```python
from build123d import *

# Parameters (mm, degrees)
SKETCH_1_W          = 35.7
SKETCH_1_H          = 25
EXTRUDE_1_DEPTH     = 1
SKETCH_2_W          = 48
SKETCH_2_H          = 14
EXTRUDE_2_DEPTH     = 57.5
FILLET_1_R          = 3
FILLET_2_R          = 5
CHAMFER_1_SIZE      = 5
HOLE_WIZARD_M3_1_D  = 3.2
CUT_EXTRUDE_START   = -15
CUT_EXTRUDE_1_DEPTH = 15
SKETCH_6_W          = 2
SKETCH_6_H          = 2
EXTRUDE_3_DEPTH     = 8
SKETCH_7_W          = 2
SKETCH_7_H          = 2
SKETCH_7_W_2        = 0.8
SKETCH_7_H_2        = 0.8
CUT_EXTRUDE_2_DEPTH = 6


with BuildPart() as part:
    # 草图1 → 凸台-拉伸1 (new body)
    with BuildSketch(Plane(origin=(0, 0, 0), x_dir=(1, 0, 0), z_dir=(0, 1, 0))):
        Rectangle(SKETCH_1_W, SKETCH_1_H)
    extrude(amount=EXTRUDE_1_DEPTH)

    # 草图2 → 凸台-拉伸2 (add)
    with BuildSketch(Plane(origin=(0, 1, 0), x_dir=(1, 0, 0), z_dir=(0, 1, 0))):
        Rectangle(SKETCH_2_W, SKETCH_2_H)
    extrude(amount=EXTRUDE_2_DEPTH)

    # 圆角1
    fillet_1_edges = [part.edges().sort_by_distance(p)[0] for p in [
        (-24, 29.75, -7),
        (24, 29.75, -7),
    ]]
    fillet(fillet_1_edges, radius=FILLET_1_R)

    # 圆角2
    fillet_2_edges = [part.edges().sort_by_distance(p)[0] for p in [
        (-24, 29.75, 7),
        (24, 29.75, 7),
    ]]
    fillet(fillet_2_edges, radius=FILLET_2_R)

    # 倒角1
    chamfer_1_edges = [part.edges().sort_by_distance(p)[0] for p in [
        (17.85, 0.5, 12.5),
        (-17.85, 0.5, 12.5),
    ]]
    chamfer(chamfer_1_edges, length=CHAMFER_1_SIZE)

    # M3 间隙孔1 (through all)
    with Locations(Plane(origin=(0, 0, 0), x_dir=(-1, 0, 0), z_dir=(0, -1, 0))):
        with Locations((0, 9.65), (-12.5, -9.65), (12.5, -9.65)):
            Hole(HOLE_WIZARD_M3_1_D / 2)

    # 草图5 → 切除-拉伸1 (cut)
    with BuildSketch(Plane.XZ.offset(-1).offset(CUT_EXTRUDE_START)):
        with BuildLine():
            Line((-24, 2), (-24, -4))
            ThreePointArc((-24, -4), (-23.121320344, -6.121320344), (-21, -7))
            Line((-21, -7), (21, -7))
            ThreePointArc((21, -7), (23.121320344, -6.121320344), (24, -4))
            Line((24, -4), (24, 2))
            ThreePointArc((24, 2), (22.535533906, 5.535533906), (19, 7))
            Line((19, 7), (-19, 7))
            ThreePointArc((-19, 7), (-22.535533906, 5.535533906), (-24, 2))
        make_face()
        with BuildLine():
            Line((-22, 2), (-22, -4))
            ThreePointArc((-22, -4), (-21.707106781, -4.707106781), (-21, -5))
            Line((-21, -5), (21, -5))
            ThreePointArc((21, -5), (21.707106781, -4.707106781), (22, -4))
            Line((22, -4), (22, 2))
            ThreePointArc((22, 2), (21.121320344, 4.121320344), (19, 5))
            Line((19, 5), (-19, 5))
            ThreePointArc((-19, 5), (-21.121320344, 4.121320344), (-22, 2))
        make_face(mode=Mode.SUBTRACT)
    extrude(amount=CUT_EXTRUDE_1_DEPTH, mode=Mode.SUBTRACT)

    # 草图6 → 凸台-拉伸3 (add)
    with BuildSketch(Plane(origin=(0, 1, 0), x_dir=(1, 0, 0), z_dir=(0, 1, 0))):
        with Locations((1.25, -9.65)):
            Rectangle(SKETCH_6_W, SKETCH_6_H)
        with Locations((-1.25, -9.65)):
            Rectangle(SKETCH_6_W, SKETCH_6_H)
        with Locations((-3.75, -9.65)):
            Rectangle(SKETCH_6_W, SKETCH_6_H)
        with Locations((-6.25, -9.65)):
            Rectangle(SKETCH_6_W, SKETCH_6_H)
        with Locations((6.25, -9.65)):
            Rectangle(SKETCH_6_W, SKETCH_6_H)
        with Locations((3.75, -9.65)):
            Rectangle(SKETCH_6_W, SKETCH_6_H)
    extrude(amount=EXTRUDE_3_DEPTH)

    # 草图7 → 切除-拉伸2 (cut)
    # profile 1 of 6: a face of its own
    with BuildSketch(Plane(origin=(0, 9, 0), x_dir=(1, 0, 0), z_dir=(0, 1, 0))):
        with Locations((-6.25, -9.65)):
            Rectangle(SKETCH_7_W, SKETCH_7_H)
        with Locations((-6.25, -9.65)):
            Rectangle(SKETCH_7_W_2, SKETCH_7_H_2, mode=Mode.SUBTRACT)
    # profile 2 of 6: a face of its own
    with BuildSketch(Plane(origin=(0, 9, 0), x_dir=(1, 0, 0), z_dir=(0, 1, 0))):
        with Locations((6.25, -9.65)):
            Rectangle(SKETCH_7_W, SKETCH_7_H)
        with Locations((6.25, -9.65)):
            Rectangle(SKETCH_7_W_2, SKETCH_7_H_2, mode=Mode.SUBTRACT)
    # profile 3 of 6: a face of its own
    with BuildSketch(Plane(origin=(0, 9, 0), x_dir=(1, 0, 0), z_dir=(0, 1, 0))):
        with Locations((3.75, -9.65)):
            Rectangle(SKETCH_7_W, SKETCH_7_H)
        with Locations((3.75, -9.65)):
            Rectangle(SKETCH_7_W_2, SKETCH_7_H_2, mode=Mode.SUBTRACT)
    # profile 4 of 6: a face of its own
    with BuildSketch(Plane(origin=(0, 9, 0), x_dir=(1, 0, 0), z_dir=(0, 1, 0))):
        with Locations((1.25, -9.65)):
            Rectangle(SKETCH_7_W, SKETCH_7_H)
        with Locations((1.25, -9.65)):
            Rectangle(SKETCH_7_W_2, SKETCH_7_H_2, mode=Mode.SUBTRACT)
    # profile 5 of 6: a face of its own
    with BuildSketch(Plane(origin=(0, 9, 0), x_dir=(1, 0, 0), z_dir=(0, 1, 0))):
        with Locations((-1.25, -9.65)):
            Rectangle(SKETCH_7_W, SKETCH_7_H)
        with Locations((-1.25, -9.65)):
            Rectangle(SKETCH_7_W_2, SKETCH_7_H_2, mode=Mode.SUBTRACT)
    # profile 6 of 6: a face of its own
    with BuildSketch(Plane(origin=(0, 9, 0), x_dir=(1, 0, 0), z_dir=(0, 1, 0))):
        with Locations((-3.75, -9.65)):
            Rectangle(SKETCH_7_W, SKETCH_7_H)
        with Locations((-3.75, -9.65)):
            Rectangle(SKETCH_7_W_2, SKETCH_7_H_2, mode=Mode.SUBTRACT)
    extrude(amount=-CUT_EXTRUDE_2_DEPTH, mode=Mode.SUBTRACT)


solid = part.part
```
Geometry: final body of the model. Coordinates: model frame, mm. A direction names the side the tool comes from. Round coordinates to 2 decimals unless told otherwise and drop trailing zeros. Order: outer loops, then holes, each group sorted by start corner. A loop starts at its lowest first (then second) coordinate and runs counter-clockwise, first axis right, second up. Notation, with made-up numbers: (88.25, 43) -> (147.25, 43) arc R20 ccw to (147.25, 66) -> close; hole circle Ø5 at (-28, 80). An arc over 180 degrees is marked (long way). Use CSV: the item, a comma, the result in double quotes. Start each with the question number.
1) Section A-A (z = -9.65). Return the cut outline in (x, y).
2) First-contact query: pin 1 Ø6 at (y, z) = (6, 5) entering from -X; pin 2 Ø8 at (y, z) = (20, -5) entering from -X; pin 3 Ø5 at (y, z) = (21, -8.5) entering from +X; pin 4 Ø1.5 at (x, y) = (12, 24.5) entering from -Z. Flat tips, straight axial feed; report the tip coordinate or a pass-through.
3) Section B-B (y = 20). Return the cut outline in (x, z), and give its area (3 significant figures).
4) Section C-C (x = 16.5). Return the cut outline in (y, z).
5) Material intervals for line 1 along Z through (x, y) = (12.5, 0.6); line 2 along X through (y, z) = (0.45, -9.65); line 3 along X through (y, z) = (0.2, 9.65), sorted ascending. Write a range as from..to.
6) Set-up query: faces 1 (the face through (20, 1, 0)), 2 (the face through (0, 37, -7)), 3 (the face through (0, 9, -5)), 4 (the face through (4, 2, 10.65)), 5 (the face through (-20, 1, 0)). Return all of +Z, -Z, +X, -X, +Y, -Y with unobstructed straight access to the full face (end or side cutting, diameter ignored); none if empty.
7) Draft query along Z for faces 6 (the face through (6, 2, 8.65)), 7 (the face through (15.39, 0.49, 9.96)), 8 (the face through (2.25, 2, 10)). Return one class per face: +Z half, -Z half, draft (parallel to the pull), parting line (faces both ways), or undercut.
Returned:
1,outline,"(-17.85, 0) -> (-1.6, 0) -> (-1.6, 1) -> (-17.85, 1) -> close; (1.6, 0) -> (17.85, 0) -> (17.85, 1) -> (1.6, 1) -> close"
2,pin 1,"stops at x = -22"
2,pin 2,"stops at x = -24"
2,pin 3,"stops at x = 23.24"
2,pin 4,"stops at z = -7"
3,outline,"(-24, -4) arc R3 ccw to (-21, -7) -> (21, -7) arc R3 ccw to (24, -4) -> (24, 2) arc R5 ccw to (19, 7) -> (-19, 7) arc R5 ccw to (-24, 2) -> close"
3,area,"657 mm²"
4,outline,"(0, -12.5) -> (1, -12.5) -> (1, -5) -> (16, -5) -> (16, -7) -> (58.5, -7) -> (58.5, 7) -> (16, 7) -> (16, 5) -> (1, 5) -> (1, 8.85) -> (0, 8.85) -> close"
5,line 1,"z = -12.5..8.05, 11.25..12.5"
5,line 2,"x = -17.85..-1.6, 1.6..17.85"
5,line 3,"x = -15.7..-14.1, -10.9..10.9, 14.1..15.7"
6,face 1,"+Z, -Z, +X, -Y"
6,face 2,"-Z, +X, -X, +Y"
6,face 3,"-Z, +X, -X"
6,face 4,"+Z, +X, -X, +Y"
6,face 5,"+Z, -Z, -X, -Y"
7,face 6,"undercut"
7,face 7,"+Z half"
7,face 8,"draft"
